Model file for the job. Use its own axes, mm. A direction names the side the tool comes from. Give positions to 0.01 mm unless a question says otherwise; leave off trailing zeros. Order: outer loops, then holes, each group sorted by start corner. A loop starts at its lowest first (then second) coordinate and runs counter-clockwise, first axis right, second up. Notation, with made-up numbers: M 58.5,-39 L 67.5,-39 A16 cw 67.5,-19 Z; hole C 68.5,42.25 d1. An arc over 180 degrees is marked long. Return JSON: item names as keys, results as strings. Group by question number.
1. Wall check: probe 1 along Y at (x, z) = (-29.5, 0.9); probe 2 along Y at (x, z) = (15, 0.25); probe 3 along Y at (x, z) = (20, 0.1). Give the ranges that are in metal, low to high. Write a range as [from, to].
2. Slice it at A-A on x = -23. List the corners of the cut face in (y, z), then the cut area to 3 significant figures.
3. Slice it at C-C on z = 0.55. List the corners of the cut face in (x, y).
4. 3-axis set-ups, long thin cutter, end or side, ignore diameter. For faces 5 (the face through (-1, -20, 1)), 6 (the face through (14, 2.07, 1)): which of +Z, -Z, +X, -X, +Y, -Y reach the whole face in a straight line?
5. Slice it at D-D on y = 0. List the corners of the cut face in (x, z), then the cut area to 3 significant figures.
6. Two-plate mould, pull along Y, no slides. Class faces 1 (the face through (-39.14, -19.1, 0.81)), 2 (the face through (-24, -12.05, 1)), 3 (the face through (-12.95, 10.05, 0.79)), 4 (the face through (-1, 20, 1)): released by +Y, released by -Y, zero draft, split by the parting line, or undercut.
7. Pin check, flat tip, straight feed: pin 1 (5 mm diameter, centred on x = -24.5, y = 8.5, fed in from -Z). Stop position of the tip, or through.
8. Slice it at B-B on x = 12. List the corners of the cut face in (y, z), then the cut area to 3 significant figures.
from build123d import *

# Parameters (mm, degrees)
SKETCH1_W           = 80
SKETCH1_H           = 40
BOSS_EXTRUDE1_DEPTH = 1.6
FILLET1_R           = 3


with BuildPart() as part:
    # Sketch1 → Boss-Extrude1 (new body)
    with BuildSketch(Plane.XY):
        Rectangle(SKETCH1_W, SKETCH1_H)
        with BuildLine():
            Line((-15, 7.95), (-33, 7.95))
            ThreePointArc((-33, 7.95), (-35.05, 10), (-33, 12.05))
            Line((-33, 12.05), (-15, 12.05))
            ThreePointArc((-15, 12.05), (-12.95, 10), (-15, 7.95))
        make_face(mode=Mode.SUBTRACT)
        with BuildLine():
            Line((-15, -7.95), (-33, -7.95))
            ThreePointArc((-33, -7.95), (-35.05, -10), (-33, -12.05))
            Line((-33, -12.05), (-15, -12.05))
            ThreePointArc((-15, -12.05), (-12.95, -10), (-15, -7.95))
        make_face(mode=Mode.SUBTRACT)
        with BuildLine():
            Line((8.9, 2.07), (18.9, 2.07))
            ThreePointArc((18.9, 2.07), (20.97, 0), (18.9, -2.07))
            Line((18.9, -2.07), (8.9, -2.07))
            ThreePointArc((8.9, -2.07), (6.83, 0), (8.9, 2.07))
        make_face(mode=Mode.SUBTRACT)
    extrude(amount=BOSS_EXTRUDE1_DEPTH)

    # Fillet1
    fillet1_edges = [part.edges().sort_by_distance(p)[0] for p in [
        (40, -20, 0.8),
        (-40, -20, 0.8),
        (-40, 20, 0.8),
        (40, 20, 0.8),
    ]]
    fillet(fillet1_edges, radius=FILLET1_R)


solid = part.part
Result:
{
 "1": {"probe 1": "y = [-20, -12.05], [-7.95, 7.95], [12.05, 20]", "probe 2": "y = [-20, -2.07], [2.07, 20]", "probe 3": "y = [-20, -1.75], [1.75, 20]"},
 "2": {"outline": "M -20,0 L -12.05,0 L -12.05,1.6 L -20,1.6 Z; M -7.95,0 L 7.95,0 L 7.95,1.6 L -7.95,1.6 Z; M 12.05,0 L 20,0 L 20,1.6 L 12.05,1.6 Z", "area": "50.9 mm2"},
 "3": {"outline": "M -40,-17 A3 ccw -37,-20 L 37,-20 A3 ccw 40,-17 L 40,17 A3 ccw 37,20 L -37,20 A3 ccw -40,17 Z; hole M -33,-12.05 L -15,-12.05 A2.05 ccw -15,-7.95 L -33,-7.95 A2.05 ccw Z; hole M -33,7.95 L -15,7.95 A2.05 ccw -15,12.05 L -33,12.05 A2.05 ccw Z; hole M 8.9,-2.07 L 18.9,-2.07 A2.07 ccw 18.9,2.07 L 8.9,2.07 A2.07 ccw Z"},
 "4": {"face 5": "+Z, -Z, +X, -X, -Y", "face 6": "+Z, -Z"},
 "5": {"outline": "M -40,0 L 6.83,0 L 6.83,1.6 L -40,1.6 Z; M 20.97,0 L 40,0 L 40,1.6 L 20.97,1.6 Z", "area": "105 mm2"},
 "6": {"face 1": "released by -Y", "face 2": "undercut", "face 3": "undercut", "face 4": "released by +Y"},
 "7": {"pin 1": "stops at z = 0"},
 "8": {"outline": "M -20,0 L -2.07,0 L -2.07,1.6 L -20,1.6 Z; M 2.07,0 L 20,0 L 20,1.6 L 2.07,1.6 Z", "area": "57.4 mm2"}
}
